```python
from build123d import *

# Parameters (mm, degrees)
F0_W     = 38.1
F0_H     = 38.1
F1_DEPTH = 0.79375
F2_W     = 38.1
F2_H     = 38.1
F2_W_2   = 34.925
F2_H_2   = 34.925
F3_DEPTH = 5.08
F4_W     = 9.0528408943
F4_H     = 1.27
F5_DEPTH = 4.445
F4_W_2   = 1.27
F4_H_2   = 10.3092815826
F4_R     = 1.27
F4_W_3   = 2.7661539333
F4_H_3   = 1.0710589232
F4_H_4   = 5.6106120447
F4_W_4   = 1.712341144
F6_DEPTH = 4.445
F7_DEPTH = 4.445
F8_DEPTH = 0.396875


with BuildPart() as f1:
    # F0 (on Top) → F1 (new body)
    with BuildSketch(Plane.XY):
        with Locations((0.4642736167, -0.8399097333)):
            Rectangle(F0_W, F0_H)
    extrude(amount=F1_DEPTH)

    # F2 (on face) → F3 (join)
    with BuildSketch(Plane.XY.offset(0.79375)):
        with Locations((0.4642736167, -0.8399097333)):
            Rectangle(F2_W, F2_H)
        with Locations((0.4642736167, -0.8399097333)):
            Rectangle(F2_W_2, F2_H_2, mode=Mode.SUBTRACT)
    extrude(amount=F3_DEPTH)

    # F4 (on face) → F5 (join)
    with BuildSketch(Plane.XY.offset(0.79375)):
        Polygon((-11.9182263833, 11.5425902667), (-11.9182263833, -18.3024097333), (-10.6482263833, -18.3024097333), (-10.6482263833, -8.8111795485), (-6.8751736544, -8.8111795485), (-6.8751736544, -7.5411795485), (-10.6482263833, -7.5411795485), (-10.6482263833, -2.2284686565), (6.4967736167, -2.2284686565), (6.4967736167, -11.2619977444), (7.7667736167, -11.2619977444), (7.7667736167, -2.2284686565), (12.8467736167, -2.2284686565), (12.8467736167, -0.9584686565), (-10.6482263833, -0.9584686565), (-10.6482263833, 10.2725902667), (1.2241147607, 10.2725902667), (1.2241147607, 4.1215313435), (2.4941147607, 4.1215313435), (5.0006196834, 4.1215313435), (5.0006196834, 5.3915313435), (2.4941147607, 5.3915313435), (2.4941147607, 10.2725902667), (2.4941147607, 11.5425902667), (-10.6482263833, 11.5425902667), align=None)
        with Locations((13.4003531695, 10.9075902667)):
            Rectangle(F4_W, F4_H)
    extrude(amount=F5_DEPTH)

    # F4 (on face) → F6 (join)
    with BuildSketch(Plane.XY.offset(0.79375)):
        Polygon((-11.9182263833, 11.5425902667), (-11.9182263833, -18.3024097333), (-10.6482263833, -18.3024097333), (-10.6482263833, -8.8111795485), (-6.8751736544, -8.8111795485), (-6.8751736544, -7.5411795485), (-10.6482263833, -7.5411795485), (-10.6482263833, -2.2284686565), (6.4967736167, -2.2284686565), (6.4967736167, -11.2619977444), (7.7667736167, -11.2619977444), (7.7667736167, -2.2284686565), (12.8467736167, -2.2284686565), (12.8467736167, -0.9584686565), (-10.6482263833, -0.9584686565), (-10.6482263833, 10.2725902667), (1.2241147607, 10.2725902667), (1.2241147607, 4.1215313435), (2.4941147607, 4.1215313435), (5.0006196834, 4.1215313435), (5.0006196834, 5.3915313435), (2.4941147607, 5.3915313435), (2.4941147607, 10.2725902667), (2.4941147607, 11.5425902667), (-10.6482263833, 11.5425902667), align=None)
        with Locations((13.4003531695, 10.9075902667)):
            Rectangle(F4_W, F4_H)
        with Locations((13.4817736167, -13.147768942)):
            Rectangle(F4_W_2, F4_H_2)
        with Locations((-14.4582263833, -16.0732418299)):
            Circle(F4_R)
        with Locations((11.46369665, 4.6570608051)):
            Rectangle(F4_W_3, F4_H_3)
        with Locations((-5.5682263833, -15.497103711)):
            Rectangle(F4_W_2, F4_H_4)
        Polygon((0.1467736167, -18.3024097333), (1.4167736167, -18.3024097333), (1.4167736167, -7.5411795485), (0.1467736167, -7.5411795485), (-1.7951736544, -7.5411795485), (-1.7951736544, -8.8111795485), (0.1467736167, -8.8111795485), align=None)
        with Locations((-4.7120558113, 4.6570608051)):
            Rectangle(F4_W_4, F4_H_3)
        with Locations((-2.3637847044, -15.662971884)):
            Circle(F4_R)
    extrude(amount=F6_DEPTH)

    # F7 (cut): faces of the model
    f7_faces = [f1.faces().sort_by_distance(p)[0] for p in [
        (-14.4582263833, -16.0732418299, 5.23875),
        (-2.3637847044, -15.662971884, 5.23875),
    ]]
    extrude(f7_faces, amount=-F7_DEPTH, mode=Mode.SUBTRACT)

    # F4 (on face) → F8 (cut)
    with BuildSketch(Plane.XY.offset(0.79375)):
        with Locations((-14.4582263833, -16.0732418299)):
            Circle(F4_R)
        with Locations((-2.3637847044, -15.662971884)):
            Circle(F4_R)
    extrude(amount=-F8_DEPTH, mode=Mode.SUBTRACT)


solid = f1.part
```
Work out the finished part from the listing and answer in its coordinate system (mm). Give positions to 0.01 mm unless a question says otherwise; leave off trailing zeros. Loops run counter-clockwise (first coordinate to the right, second up) from the corner with the lowest first, then second, coordinate; pieces in that order, holes last. Notation, with made-up numbers: (-39, 21) - (1, 21) arc R28 cw to (1, 40) - close; hole circle Ø7 at (87.25, 34). An arc over 180 degrees is marked (long way). Use CSV: the item, a comma, the result in double quotes. Start each with the question number.
(1) Find section C-C, the plane x = 6. Determine the outline of the cut face in (y, z), plus the area to 3 significant figures.
(2) Determine the mould class of faces 1 (the face through (-18.586, -1, 3)), 2 (the face through (0, 18.21, 3)), 3 (the face through (-10.648, -5, 3)) for opening direction X: released by +X, released by -X, zero draft, split by the parting line, or undercut.
(3) Find section D-D, the plane y = 6. Determine the outline of the cut face in (x, z).
(4) Find section B-B, the plane y = 13. Determine the outline of the cut face in (x, z), plus the area to 3 significant figures.
(5) Each of these flat-tipped pins is pushed along its axis until it touches: pin 1 (2 mm diameter, centred on x = -14.46, y = -16.07, fed in from +Z); pin 2 (1.4 mm diameter, centred on x = 13.5, y = -13, fed in from +Z). Where does it stop, or does it pass through?
(6) Find the intervals of material crossed by L1, parallel to Y at x = 15, z = 2.05; L2, parallel to Y at x = 7, z = 1.9; L3, parallel to X at y = -6, z = 3.4, in increasing order.
(7) Find section A-A, the plane z = 2.8. Count the separate pieces of the cut face and the enclosed holes in it, plus the area to 3 significant figures.
Results found:
1,outline,"(-19.89, 0) - (18.21, 0) - (18.21, 5.87) - (16.62, 5.87) - (16.62, 0.79) - (-0.96, 0.79) - (-0.96, 5.24) - (-2.23, 5.24) - (-2.23, 0.79) - (-18.3, 0.79) - (-18.3, 5.87) - (-19.89, 5.87) - close"
1,area,"52.0 mm^2"
2,face 1,"released by -X"
2,face 2,"zero draft"
2,face 3,"undercut"
3,outline,"(-18.59, 0) - (19.51, 0) - (19.51, 5.87) - (17.93, 5.87) - (17.93, 0.79) - (2.49, 0.79) - (2.49, 5.24) - (1.22, 5.24) - (1.22, 0.79) - (-10.65, 0.79) - (-10.65, 5.24) - (-11.92, 5.24) - (-11.92, 0.79) - (-17, 0.79) - (-17, 5.87) - (-18.59, 5.87) - close"
4,outline,"(-18.59, 0) - (19.51, 0) - (19.51, 5.87) - (17.93, 5.87) - (17.93, 0.79) - (-17, 0.79) - (-17, 5.87) - (-18.59, 5.87) - close"
4,area,"46.4 mm^2"
5,pin 1,"z = 0.4"
5,pin 2,"z = 5.24"
6,L1,"-19.89 to -18.3, 10.27 to 11.54, 16.62 to 18.21"
6,L2,"-19.89 to -18.3, -11.26 to -0.96, 16.62 to 18.21"
6,L3,"-18.59 to -17, -11.92 to -10.65, 6.5 to 7.77, 17.93 to 19.51"
7,separate pieces,"3"
7,enclosed holes,"1"
7,area,"396 mm^2"
